Autodesk Inventor part; units mm, degrees
ref_plane "Work Plane9" through (-30.1625, 0, 451.8) normal (0.2588, 0, 0.9659) x (0, 1, 0)
ref_plane "Work Plane10" through (0, 30.1625, 0) normal (0, 1, 0) x (-1, 0, 0)
ref_plane "Work Plane11" through (0, -30.1625, 0) normal (0, -1, 0) x (1, 0, 0)
sketch "Sketch1" plane through (0, 0, 0) normal (0, 0, 1) x (1, 0, 0)
  circle A0 centre (0, 0) radius 30.1625
  circle A1 centre (0, 0) radius 26.2509
  dimension "d0" = 60.325
  dimension "d2" = 3.9116
extrude "Extrusion1" add sketch "Sketch1" along normal blind 451.8
sketch "Sketch18" plane through (0, 0, 451.8) normal (0, 0, 1) x (1, 0, 0)
  circle A0 centre (0, 0) radius 26.2509
  circle A1 centre (0, 0) radius 30.1625
  point P0 (-30.1625, 0)
ref_plane "Work Plane9" through (-30.1625, 0, 451.8) normal (0.2588, 0, 0.9659) x (0, 1, 0)
sketch "Sketch19" plane through (-30.1625, 0, 451.8) normal (0.2588, 0, 0.9659) x (0, 1, 0)
  line L0 (-31.6137, -94.9476) -> (64.4261, -94.9476)
  line L1 (64.4261, -94.9476) -> (64.4261, 6.6524)
  line L2 (64.4261, 6.6524) -> (-31.6137, 6.6524)
  line L3 (-31.6137, 6.6524) -> (-31.6137, -94.9476)
  point P0 (0, -146.0692)
  dimension "d61" = 101.6
extrude "Extrusion11" cut sketch "Sketch19" along normal blind 25.4
sketch "Sketch20" plane through (0, 0, 0) normal (0, 0, -1) x (-1, 0, 0)
  circle A0 centre (0, 0) radius 26.2509
  circle A1 centre (0, 0) radius 30.1625
  point P0 (0, 30.1625)
  point P1 (0, -30.1625)
ref_plane "Work Plane10" through (0, 30.1625, 0) normal (0, 1, 0) x (-1, 0, 0)
ref_plane "Work Plane11" through (0, -30.1625, 0) normal (0, -1, 0) x (1, 0, 0)
sketch "Sketch21" plane through (0, 30.1625, 0) normal (0, 1, 0) x (-1, 0, 0)
  line L0 (-3.1444, 451.8) -> (6.8556, 451.8)
  line L1 (6.8556, 451.8) -> (6.8556, 351.8)
  line L2 (6.8556, 351.8) -> (-3.1444, 351.8)
  line L3 (-3.1444, 351.8) -> (-3.1444, 451.8)
  line L4 (1.8556, 451.8) -> (1.8556, 351.8) construction
  point P0 (0, 0)
  dimension "d64" = 10
  dimension "d65" = 100
  dimension "d82" = 351.8
extrude "flat1" cut sketch "Sketch21" against normal blind 0.254
sketch "Sketch22" plane through (0, -30.1625, 0) normal (0, -1, 0) x (1, 0, 0)
  line L0 (-3.1568, 351.8) -> (6.8432, 351.8)
  line L1 (6.8432, 351.8) -> (6.8432, 451.8)
  line L2 (6.8432, 451.8) -> (-3.1568, 451.8)
  line L3 (-3.1568, 451.8) -> (-3.1568, 351.8)
  line L4 (1.8432, 451.8) -> (1.8432, 351.8) construction
  point P0 (0, 0)
  dimension "d68" = 10
  dimension "d69" = 100
  dimension "d83" = 351.8
extrude "flat2" cut sketch "Sketch22" against normal blind 0.254
sketch "Sketch23" plane through (0, -29.9085, 0) normal (0, -1, 0) x (1, 0, 0)
  circle A0 centre (0, 424.5638) radius 1.4603
  circle A1 centre (0, 384.5638) radius 1.4603
  point P0 (-3.1568, 444.5638)
  point P1 (0, 0)
  dimension "d73" = 40
  dimension "d74" = 20
hole "Hole1" at (0, -29.9085, 424.5638) at (0, -29.9085, 384.5638) direction (0, 1, 0) diameter 3.175 end through all
properties part number "2r2scs" material "PVC-Piping"
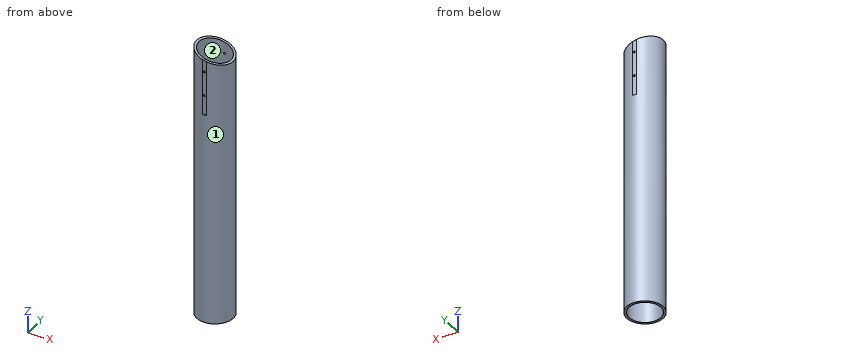
Verification items for the finished model (mm, model axes). Face numbers are marked on the shaded views. Give positions to 0.01 mm unless a question says otherwise; leave off trailing zeros. Order: outer loops, then holes, each group sorted by start corner. A loop starts at its lowest first (then second) coordinate and runs counter-clockwise, first axis right, second up. Notation, with made-up numbers: M 39,28.25 L 77,28.25 A11 cw 77,40.25 Z; hole C 60,15 d3. An arc over 180 degrees is marked long. Return JSON: item names as keys, results as strings. Group by question number.
1) Section check D-D on z = 253. Record the cut outline in (x, y) (1 decimal).
2) Scan lines: line 1 (X direction, y = 0, z = 259); line 2 (Z direction, x = 0, y = -27.25); line 3 (Y direction, x = -0.5, z = 396). Record each from-to range of solid material in increasing order.
3) Mould release check, pull along X, two halves, no side actions. Record for the marked faces 1 and 2: pulls with the +X half, pulls with the -X half, needs draft (parallel to the pull), parting line crosses it, or undercut.
4) Section check A-A on y = -9. Record the cut outline in (x, z), and give its area (3 significant figures).
5) Go/stop test with flat-tipped pins: pin 1 Ø10 at (x, z) = (-18, 385) entering from +Y; pin 2 Ø12 at (y, z) = (23, 373) entering from -X; pin 3 Ø5 at (x, z) = (0, 384.56) entering from -Y; pin 4 Ø3 at (x, z) = (0, 424.56) entering from -Y. Record where each tip stops, or that it passes through.
6) Section check C-C on x = -22.5. Record the cut outline in (y, z).
Answer block:
{
 "1": {"outline": "C 0,0 d60.3; hole C 0,0 d52.5"},
 "2": {"line 1": "x = -30.16 to -26.25, 26.25 to 30.16", "line 2": "z = 0 to 382.98, 386.15 to 422.98, 426.15 to 443.72", "line 3": "y = -29.91 to -26.25, 26.25 to 29.91"},
 "3": {"face 1": "parting line crosses it", "face 2": "undercut"},
 "4": {"outline": "M -28.79,0 L -24.66,0 L -24.66,450.32 L -28.79,451.43 Z; M 24.66,0 L 28.79,0 L 28.79,436 L 24.66,437.11 Z", "area": "3,660 mm^2"},
 "5": {"pin 1": "stops at y = 27.22", "pin 2": "stops at x = -24.92", "pin 3": "stops at y = -29.91", "pin 4": "passes through"},
 "6": {"outline": "M -20.09,0 L -13.52,0 L -13.52,449.74 L -20.09,449.74 Z; M 13.52,0 L 20.09,0 L 20.09,449.74 L 13.52,449.74 Z"}
}
